from build123d import *

# Parameters (mm, degrees)
EXTRUDE_1_DEPTH     = 30
FILLET_1_R          = 8
SKETCH_4_R          = 1.65
CUT_EXTRUDE_1_DEPTH = 10
SKETCH_5_R          = 1.65
CUT_EXTRUDE_2_DEPTH = 10
SKETCH_6_R          = 1.5
CUT_EXTRUDE_3_DEPTH = 10


with BuildPart() as part:
    # 草图1 → 凸台-拉伸1 (new body)
    with BuildSketch(Plane.XY):
        Polygon((0, 0), (29.5, 0), (29.5, -26), (25.5, -26), (25.5, -4), (0, -4), (-25.5, -4), (-25.5, -26), (-29.5, -26), (-29.5, 0), align=None)
    extrude(amount=EXTRUDE_1_DEPTH)

    # 圆角1
    fillet_1_edges = [part.edges().sort_by_distance(p)[0] for p in [
        (27.5, -26, 0),
        (-27.5, -26, 0),
        (-27.5, -26, 30),
        (27.5, -26, 30),
    ]]
    fillet(fillet_1_edges, radius=FILLET_1_R)

    # 草图4 → 切除-拉伸1 (cut)
    with BuildSketch(Plane(origin=(0, 0, 0), x_dir=(1, 0, 0), z_dir=(0, 1, 0))):
        with Locations((15, -11.5)):
            Circle(SKETCH_4_R)
        with Locations((-15, -11.5)):
            Circle(SKETCH_4_R)
    extrude(amount=-CUT_EXTRUDE_1_DEPTH, mode=Mode.SUBTRACT)

    # 草图5 → 切除-拉伸2 (cut)
    with BuildSketch(Plane.ZY.offset(29.5)):
        with Locations((15, -13)):
            Circle(SKETCH_5_R)
    extrude(amount=-CUT_EXTRUDE_2_DEPTH, mode=Mode.SUBTRACT)

    # 草图6 → 切除-拉伸3 (cut)
    with BuildSketch(Plane(origin=(29.5, 0, 0), x_dir=(0, 0, -1), z_dir=(1, 0, 0))):
        with Locations((-15, -6)):
            Circle(SKETCH_6_R)
        with Locations((-8, -13)):
            Circle(SKETCH_6_R)
        with Locations((-15, -20)):
            Circle(SKETCH_6_R)
        with Locations((-22, -13)):
            Circle(SKETCH_6_R)
    extrude(amount=-CUT_EXTRUDE_3_DEPTH, mode=Mode.SUBTRACT)


solid = part.part
Input: part model. Units: mm. Frame: model coordinates. A direction names the side the tool comes from. Coordinates: 2 decimals unless noted, no trailing zeros. Order: outer loops, then holes, each group sorted by start corner. A loop starts at its lowest first (then second) coordinate and runs counter-clockwise, first axis right, second up. Notation, with made-up numbers: M 43.5,83.5 L 55.5,83.5 A22 ccw 55.5,117.5 Z; hole C -2,7.5 d6. An arc over 180 degrees is marked long. Answer in a Markdown table with one row per item.
(1) Contact query for flat-ended pins moving along their axis: pin 1 Ø2.5 at (y, z) = (-13, 22) entering from +X; pin 2 Ø6 at (x, z) = (21.5, 12.5) entering from -Y. Output: stop coordinate, or through.
Numbers:
| item | result |
|---|---|
| pin 1 | stops at x = -25.5 |
| pin 2 | stops at y = -4 |
(2) Section query A-A, the plane y = -17. Output: boundary loops of the cut face in (x, z).
Numbers:
| item | result |
|---|---|
| outline | M -29.5,0 L -25.5,0 L -25.5,30 L -29.5,30 Z; M 25.5,0 L 29.5,0 L 29.5,30 L 25.5,30 Z |
(3) Section query C-C, the plane x = 15. Output: boundary loops of the cut face in (y, z), plus the area to 3 significant figures.
Numbers:
| item | result |
|---|---|
| outline | M -4,0 L 0,0 L 0,9.85 L -4,9.85 Z; M -4,13.15 L 0,13.15 L 0,30 L -4,30 Z |
| area | 107 mm^2 |
(4) Section query D-D, the plane y = -20. Output: boundary loops of the cut face in (x, z), plus the area to 3 significant figures.
Numbers:
| item | result |
|---|---|
| outline | M -29.5,0.25 L -25.5,0.25 L -25.5,29.75 L -29.5,29.75 Z; M 25.5,0.25 L 29.5,0.25 L 29.5,13.5 L 25.5,13.5 Z; M 25.5,16.5 L 29.5,16.5 L 29.5,29.75 L 25.5,29.75 Z |
| area | 224 mm^2 |
(5) Access query for faces 1 (the flat face through (25.5, -15, 15)), 2 (the cylindrical face through (27.53, -18.99, 16.11)), 3 (the flat face through (-27, -26, 15)). Directions: +Z, -Z, +X, -X, +Y, -Y. A direction counts if a zero-diameter tool reaches every point of the face in a straight line with its end or side. Return the directions, or none.
Numbers:
| item | result |
|---|---|
| face 1 | +Z, -Z, -Y |
| face 2 | +X |
| face 3 | +Z, -Z, +X, -X, -Y |
(6) Section query B-B, the plane z = 11.5. Output: boundary loops of the cut face in (x, y).
Numbers:
| item | result |
|---|---|
| outline | M -29.5,-26 L -25.5,-26 L -25.5,-4 L -16.65,-4 L -16.65,0 L -29.5,0 Z; M -13.35,-4 L 13.35,-4 L 13.35,0 L -13.35,0 Z; M 16.65,-4 L 25.5,-4 L 25.5,-26 L 29.5,-26 L 29.5,0 L 16.65,0 Z |
(7) Material intervals for line 1 (X direction, y = -18.75, z = 8.5); line 2 (X direction, y = -2.3, z = 11.5); line 3 (Y direction, x = 28.6, z = 15), sorted ascending. Write a range as [from, to].
Numbers:
| item | result |
|---|---|
| line 1 | x = [-29.5, -25.5], [25.5, 29.5] |
| line 2 | x = [-29.5, -16.65], [-13.35, 13.35], [16.65, 29.5] |
| line 3 | y = [-26, -21.5], [-18.5, -7.5], [-4.5, 0] |
(8) Draft query along Z for faces 4 (the flat face through (-29.5, -10, 15)), 5 (the cylindrical face through (27.472, -23.719, 27.594)), 6 (the cylindrical face through (-27.528, -13.632, 16.524)). Return one class per face: pulls with the +Z half, pulls with the -Z half, needs draft (parallel to the pull), parting line crosses it, or undercut.
Numbers:
| item | result |
|---|---|
| face 4 | needs draft |
| face 5 | pulls with the +Z half |
| face 6 | undercut |
